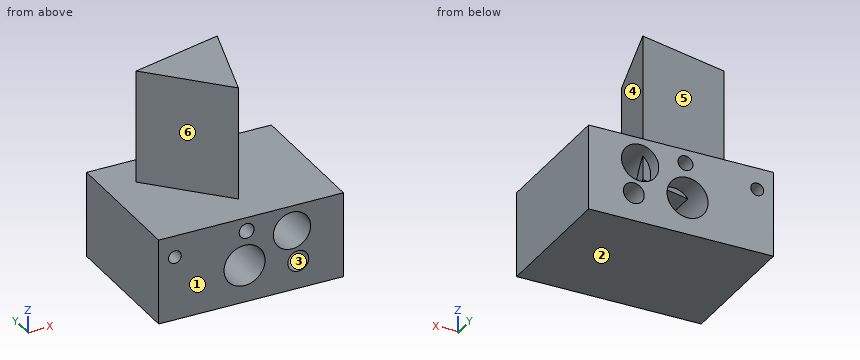
```python
from build123d import *

# Parameters (mm, degrees)
F0_W     = 118.970122
F0_H     = 54.950323
F0_R     = 13.191556
F0_R_2   = 6.719496
F0_R_3   = 4.107262
F0_R_4   = 4.798819
F0_R_5   = 12.010022
F1_DEPTH = 88.9
F3_DEPTH = 93.98


with BuildPart() as f1:
    # F0 (on Front) → F1 (new body)
    with BuildSketch(Plane.XZ):
        with Locations((20.006189, -6.268603)):
            Rectangle(F0_W, F0_H)
        with Locations((15.80747, -9.807219)):
            Circle(F0_R, mode=Mode.SUBTRACT)
        with Locations((50.417498, -15.826354)):
            Circle(F0_R_2, mode=Mode.SUBTRACT)
        with Locations((-29.035088, 7.347315)):
            Circle(F0_R_3, mode=Mode.SUBTRACT)
        with Locations((17.161777, 12.463582)):
            Circle(F0_R_4, mode=Mode.SUBTRACT)
        with Locations((46.354581, 5.09014)):
            Circle(F0_R_5, mode=Mode.SUBTRACT)
    extrude(amount=F1_DEPTH)

    # F2 (on Top) → F3 (join)
    with BuildSketch(Plane.XY):
        Polygon((23.00154, -67.576603), (40.219564, -8.440484), (-19.602828, -23.097298), align=None)
    extrude(amount=F3_DEPTH)


solid = f1.part
```
Design review of the part built by this model. Coordinates are the model's own, in mm. Face numbers are marked on the shaded views. A direction names the side the tool comes from. Coordinates: 2 decimals unless noted, no trailing zeros. Loops run counter-clockwise (first coordinate to the right, second up) from the corner with the lowest first, then second, coordinate; pieces in that order, holes last. Notation, with made-up numbers: (-22.75, -23.75) - (-9.75, -23.75) arc R12 cw to (-9.75, -19.75) - close; hole circle Ø11 at (-23.75, -21). An arc over 180 degrees is marked (long way). Use CSV: the item, a comma, the result in double quotes. Start each with the question number.
1) Wall thickness on L1, parallel to X at y = -62.5, z = 15.5; L2, parallel to X at y = -77.5, z = 13; L3, parallel to Z at x = 55.5, y = -81: over which ranges is each line inside the solid? List them lowest first. Write a range as from..to.
2) Consider section D-D on y = -76. Write out the cut boundary in (x, z), then the cut area to 3 significant figures.
3) Consider section B-B on z = -13. Write out the cut boundary in (x, y).
4) Consider section A-A on x = 52. Write out the cut boundary in (y, z), then the cut area to 3 significant figures.
5) Consider section C-C on x = 4.5. Write out the cut boundary in (y, z).
6) For pin 1 Ø7.5 at (x, z) = (17.16, 12.46) entering from -Y; pin 2 Ø10.5 at (x, z) = (-29.04, 7.35) entering from +Y; pin 3 Ø8.5 at (x, z) = (17.16, 12.46) entering from +Y; pin 4 Ø1.5 at (x, y) = (63, -75.5) entering from +Z, all flat-tipped, find the tip position at first contact; note any pin that passes through.
7) The part is to be moulded in two halves that separate along Z. For the marked faces 1, 2 and 3, say which applies: +Z half, -Z half, draft (parallel to the pull), parting line (faces both ways), or undercut.
8) Tool access review of the marked faces 4, 5 and 6: name each direction out of +Z, -Z, +X, -X, +Y, -Y from which nothing blocks a thin tool from reaching the whole face with its end or side.
Geometry says:
1,L1,"-39.48..13.45, 18.14..40.36, 52.34..79.49"
1,L2,"-39.48..12.39, 21.93..37.32, 55.39..79.49"
1,L3,"-33.74..-20.22, -11.43..-2.69, 12.87..21.21"
2,outline,"(-39.48, -33.74) - (79.49, -33.74) - (79.49, 21.21) - (-39.48, 21.21) - close; hole circle Ø8.21 at (-29.04, 7.35); hole circle Ø26.38 at (15.81, -9.81); hole circle Ø9.6 at (17.16, 12.46); hole circle Ø24.02 at (46.35, 5.09); hole circle Ø13.44 at (50.42, -15.83)"
2,area,"5,270 mm^2"
3,outline,"(-39.48, -88.9) - (3.01, -88.9) - (3.01, 0) - (-39.48, 0) - close; (28.61, -88.9) - (44.32, -88.9) - (44.32, 0) - (28.61, 0) - close; (56.51, -88.9) - (79.49, -88.9) - (79.49, 0) - (56.51, 0) - close"
4,outline,"(-88.9, -33.74) - (0, -33.74) - (0, -22.36) - (-88.9, -22.36) - close; (-88.9, -9.3) - (0, -9.3) - (0, -5.51) - (-88.9, -5.51) - close; (-88.9, 15.69) - (0, 15.69) - (0, 21.21) - (-88.9, 21.21) - close"
4,area,"1,840 mm^2"
5,outline,"(-88.9, -33.74) - (0, -33.74) - (0, -16.6) - (-88.9, -16.6) - close; (-88.9, -3.01) - (0, -3.01) - (0, 21.21) - (-17.19, 21.21) - (-17.19, 93.98) - (-48.26, 93.98) - (-48.26, 21.21) - (-88.9, 21.21) - close"
6,pin 1,"y = -65.39"
6,pin 2,"y = 0"
6,pin 3,"y = -13.05"
6,pin 4,"z = 21.21"
7,face 1,"draft"
7,face 2,"-Z half"
7,face 3,"undercut"
8,face 4,"+Z, +X, -Y"
8,face 5,"+Z, -X, +Y"
8,face 6,"+Z, -X, -Y"
